Build history of the part. All positions in model axes, mm. A direction names the side the tool comes from. Coordinates: 2 decimals unless noted, no trailing zeros. Loops run counter-clockwise (first coordinate to the right, second up) from the corner with the lowest first, then second, coordinate; pieces in that order, holes last.
Item 1: Mould opens along Y. For faces 1 (the face through (15, 7, 28)), 2 (the face through (0, 20.625, 10)), 3 (the face through (0, 0, 0.2)) say: released by +Y, released by -Y, zero draft, split by the parting line, or undercut.
Item 2: Cut at D-D (x = -17.5). List the corners of the cut face in (y, z) (3 decimals), and give its area (3 significant figures).
Item 3: Cut at A-A (z = 10.5). List the corners of the cut face in (x, y) (3 decimals).
Item 4: Drill centre lines: line 1 along Y through (x, z) = (-8.5, 19.5) (3 decimals); line 2 along Z through (x, y) = (19, -8.5); line 3 along X through (y, z) = (-12.5, 8.5). Where is each one in solid material? Low to high.
Item 5: 3-axis set-ups, long thin cutter, end or side, ignore diameter. For faces 4 (the face through (28.5, -5, 11)), 5 (the face through (-18.28, 20.87, 4.55)), 6 (the face through (3.53, 4.17, 24.45)): which of +Z, -Z, +X, -X, +Y, -Y reach the whole face in a straight line?
Item 6: Cut at B-B (x = 14.5). List the corners of the cut face in (y, z) (3 decimals), and give its area (3 significant figures).
Item 7: Cut at C-C (y = 4). List the corners of the cut face in (x, z), and give its area (3 significant figures).
Item 8: Flat gauge pins, fed straight in: pin 1 (4 mm diameter, centred on x = 17.5, z = 24, fed in from +Y); pin 2 (0.5 mm diameter, centred on x = 29, z = 11, fed in from +Y) (3 decimals); pin 3 (7 mm diameter, centred on y = -6.5, z = 12, fed in from +X). Where does each tip first touch, or does it go through?
from build123d import *

# Parameters (mm, degrees)
SKETCH1_W           = 59
SKETCH1_H           = 41.25
BOSS_EXTRUDE1_DEPTH = 21
SKETCH2_R           = 11.5
BOSS_EXTRUDE2_DEPTH = 7
SKETCH3_R           = 6.1
BOSS_EXTRUDE3_DEPTH = 0.5
SKETCH4_W           = 14.5
SKETCH4_H           = 24
CUT_EXTRUDE1_DEPTH  = 1
SKETCH5_W           = 47
SKETCH5_H           = 36.5
CUT_EXTRUDE2_DEPTH  = 0.2
SKETCH6_R           = 6
BOSS_EXTRUDE4_DEPTH = 0.5


with BuildPart() as part:
    # Sketch1 → Boss-Extrude1 (new body)
    with BuildSketch(Plane.XY):
        Rectangle(SKETCH1_W, SKETCH1_H)
    extrude(amount=BOSS_EXTRUDE1_DEPTH)

    # Sketch2 → Boss-Extrude2 (add)
    with BuildSketch(Plane.XY.offset(21)):
        with Locations(Location((14.5, 7.625, 0), (0, 0, 180))):
            Circle(SKETCH2_R)
    extrude(amount=BOSS_EXTRUDE2_DEPTH)

    # Sketch3 → Boss-Extrude3 (add)
    with BuildSketch(Plane.XY.offset(21)):
        with Locations(Location((-17, -10.625, 0), (0, 0, 180))):
            Circle(SKETCH3_R)
    extrude(amount=BOSS_EXTRUDE3_DEPTH)

    # Sketch4 → Cut-Extrude1 (cut)
    with BuildSketch(Plane(origin=(29.5, 0, 0), x_dir=(0, 0, -1), z_dir=(1, 0, 0))):
        with Locations((-10.5, -5.125)):
            Rectangle(SKETCH4_W, SKETCH4_H)
    extrude(amount=-CUT_EXTRUDE1_DEPTH, mode=Mode.SUBTRACT)

    # Sketch5 → Cut-Extrude2 (cut)
    with BuildSketch(Plane(origin=(0, 0, 0), x_dir=(-1, 0, 0), z_dir=(0, 0, -1))):
        Rectangle(SKETCH5_W, SKETCH5_H)
    extrude(amount=-CUT_EXTRUDE2_DEPTH, mode=Mode.SUBTRACT)

    # Sketch6 → Boss-Extrude4 (add)
    with BuildSketch(Plane(origin=(0, 20.625, 0), x_dir=(1, 0, 0), z_dir=(0, 1, 0))):
        with Locations((-17.5, -10.5)):
            Circle(SKETCH6_R)
    extrude(amount=BOSS_EXTRUDE4_DEPTH)


solid = part.part
Filled sheet:
1. face 1: zero draft
1. face 2: released by +Y
1. face 3: undercut
2. outline: (-20.625, 0) - (-18.25, 0) - (-18.25, 0.2) - (18.25, 0.2) - (18.25, 0) - (20.625, 0) - (20.625, 4.5) - (21.125, 4.5) - (21.125, 16.5) - (20.625, 16.5) - (20.625, 21) - (-4.546, 21) - (-4.546, 21.5) - (-16.704, 21.5) - (-16.704, 21) - (-20.625, 21) - close
2. area: 871 mm2
3. outline: (-29.5, -20.625) - (29.5, -20.625) - (29.5, -17.125) - (28.5, -17.125) - (28.5, 6.875) - (29.5, 6.875) - (29.5, 20.625) - (-11.5, 20.625) - (-11.5, 21.125) - (-23.5, 21.125) - (-23.5, 20.625) - (-29.5, 20.625) - close
4. line 1: y = -20.625 to 20.625
4. line 2: z = 0.2 to 21
4. line 3: x = -29.5 to 28.5
5. face 4: +X
5. face 5: +Y
5. face 6: +Z
6. outline: (-20.625, 0) - (-18.25, 0) - (-18.25, 0.2) - (18.25, 0.2) - (18.25, 0) - (20.625, 0) - (20.625, 21) - (19.125, 21) - (19.125, 28) - (-3.875, 28) - (-3.875, 21) - (-20.625, 21) - close
6. area: 1,020 mm2
7. outline: (-29.5, 0) - (-23.5, 0) - (-23.5, 0.2) - (23.5, 0.2) - (23.5, 0) - (29.5, 0) - (29.5, 3.25) - (28.5, 3.25) - (28.5, 17.75) - (29.5, 17.75) - (29.5, 21) - (25.41, 21) - (25.41, 28) - (3.59, 28) - (3.59, 21) - (-29.5, 21) - close
7. area: 1,370 mm2
8. pin 1: stops at y = 19.08
8. pin 2: stops at y = 20.625
8. pin 3: stops at x = 28.5
